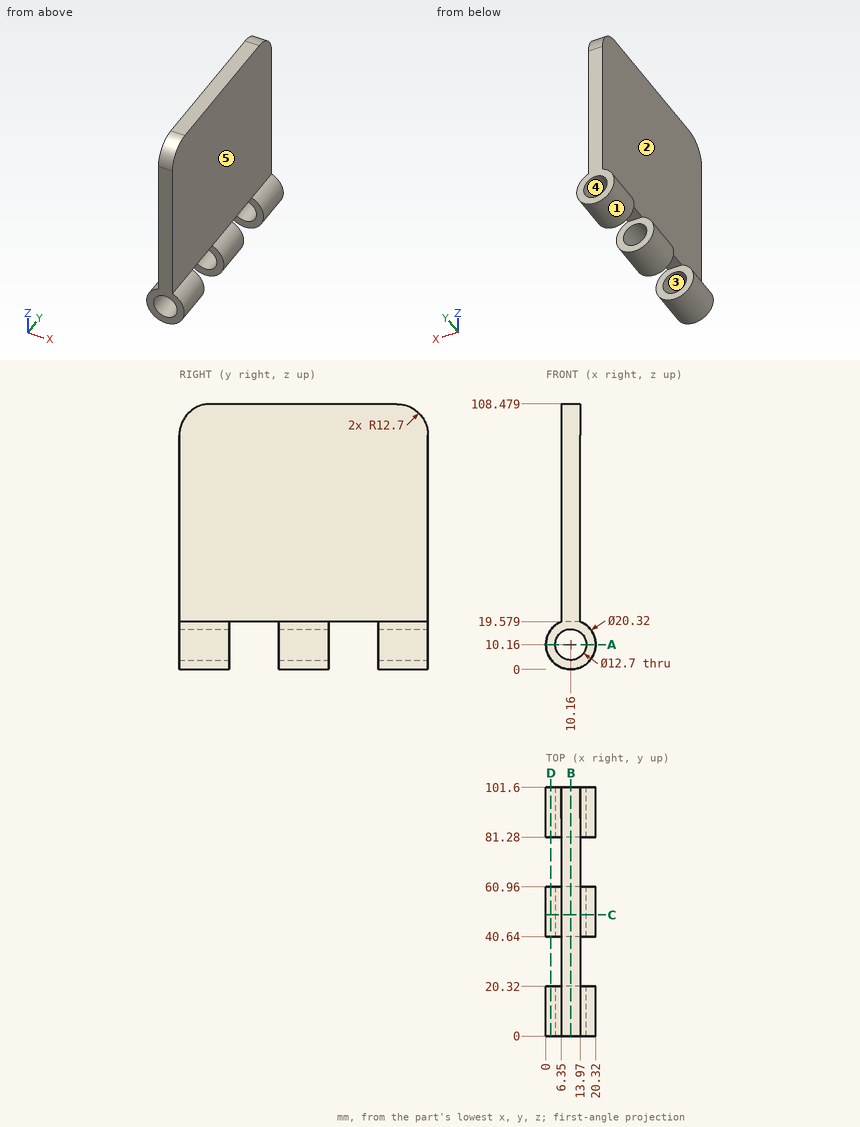
The drawing under review shows one solid part. Ordinate dimensions are in mm from its lowest x, y, z. A direction names the side the tool comes from. Give positions to 0.01 mm unless a question says otherwise; leave off trailing zeros. Loops run counter-clockwise (first coordinate to the right, second up) from the corner with the lowest first, then second, coordinate; pieces in that order, holes last. Notation, with made-up numbers: M 1,-27 L 35,-27 A25 ccw 35,-1 Z; hole C 66.25,85.25 d1. An arc over 180 degrees is marked long. Return JSON: item names as keys, results as strings. Group by question number.
Item 1: For probe 1 along Y at (x, z) = (12.75, 16.5); probe 2 along Z at (x, y) = (10.16, 52.5); probe 3 along X at (y, z) = (41, 12), list the stretches that pass through material, from the lowest coordinate up.
Item 2: We need section C-C (y = 49.5). Give the boundary of the cut face in (x, z), and give its area (3 significant figures).
Item 3: Tool access review of the marked faces 4 and 5: name each direction out of +Z, -Z, +X, -X, +Y, -Y from which nothing blocks a thin tool from reaching the whole face with its end or side.
Item 4: We need section B-B (x = 10.16). Give the boundary of the cut face in (y, z), and give its area (3 significant figures).
Item 5: Mouldability with a two-part tool opening along Z and no side actions: class the marked faces 1, 2 and 3 as released by +Z, released by -Z, zero draft, split by the parting line, or undercut.
Item 6: We need section D-D (x = 2). Give the boundary of the cut face in (y, z), and give its area (3 significant figures).
Item 7: Insertion check: pin 1 Ø1.5 at (y, z) = (52.5, 86) entering from +X; pin 2 Ø1.5 at (y, z) = (15.5, 69.5) entering from -X; pin 3 Ø3 at (x, y) = (13, 31) entering from -Z; pin 4 Ø11.5 at (x, z) = (10.16, 10.16) entering from +Y. Each pin has a flat end and moves straight along its axis. Give the tip position at first contact, or say it passes through.
Item 8: We need section A-A (z = 10.16). Give the boundary of the cut face in (x, y).
Output:
{
 "1": {"probe 1": "y = 0 to 20.32, 40.64 to 60.96, 81.28 to 101.6", "probe 2": "z = 0 to 3.81, 16.51 to 108.48", "probe 3": "x = 0.17 to 4.08, 16.24 to 20.15"},
 "2": {"outline": "M 6.35,19.58 A10.16 ccw long 13.97,19.58 L 13.97,108.48 L 6.35,108.48 Z; hole C 10.16,10.16 d12.7", "area": "871 mm^2"},
 "3": {"face 4": "+Y, -Y", "face 5": "+Z, +X, +Y, -Y"},
 "4": {"outline": "M 0,0 L 20.32,0 L 20.32,3.81 L 0,3.81 Z; M 0,16.51 L 20.32,16.51 L 20.32,19.58 L 40.64,19.58 L 40.64,16.51 L 60.96,16.51 L 60.96,19.58 L 81.28,19.58 L 81.28,16.51 L 101.6,16.51 L 101.6,95.78 A12.7 ccw 88.9,108.48 L 12.7,108.48 A12.7 ccw 0,95.78 Z; M 40.64,0 L 60.96,0 L 60.96,3.81 L 40.64,3.81 Z; M 81.28,0 L 101.6,0 L 101.6,3.81 L 81.28,3.81 Z", "area": "9,380 mm^2"},
 "5": {"face 1": "split by the parting line", "face 2": "zero draft", "face 3": "undercut"},
 "6": {"outline": "M 0,4.11 L 20.32,4.11 L 20.32,16.21 L 0,16.21 Z; M 40.64,4.11 L 60.96,4.11 L 60.96,16.21 L 40.64,16.21 Z; M 81.28,4.11 L 101.6,4.11 L 101.6,16.21 L 81.28,16.21 Z", "area": "738 mm^2"},
 "7": {"pin 1": "stops at x = 13.97", "pin 2": "stops at x = 6.35", "pin 3": "stops at z = 19.58", "pin 4": "passes through"},
 "8": {"outline": "M 0,0 L 3.81,0 L 3.81,20.32 L 0,20.32 Z; M 0,40.64 L 3.81,40.64 L 3.81,60.96 L 0,60.96 Z; M 0,81.28 L 3.81,81.28 L 3.81,101.6 L 0,101.6 Z; M 16.51,0 L 20.32,0 L 20.32,20.32 L 16.51,20.32 Z; M 16.51,40.64 L 20.32,40.64 L 20.32,60.96 L 16.51,60.96 Z; M 16.51,81.28 L 20.32,81.28 L 20.32,101.6 L 16.51,101.6 Z"}
}
